Input: part model. Units: mm. Frame: model coordinates. Face numbers are marked on the shaded views. A direction names the side the tool comes from. Coordinates: 2 decimals unless noted, no trailing zeros. Loops run counter-clockwise (first coordinate to the right, second up) from the corner with the lowest first, then second, coordinate; pieces in that order, holes last.
(1) Contact query for flat-ended pins moving along their axis: P1, Ø1.5, axis at y = -12.5, z = 2, coming from the -X side; P2, Ø1, axis at y = 3, z = 1.5, coming from the -X side. Output: stop coordinate, or through.
(2) Mould query, pull axis X, two halves, no side actions, for the marked faces 1, 2, 3 and 4. Classes: released by +X, released by -X, zero draft, split by the parting line, or undercut.
(3) Section A-A, the plane z = 0.8. Return loops of the section in (x, y), then the cut area to 3 significant figures.
(4) Set-up query: the marked faces 5 and 6. Return all of +Z, -Z, +X, -X, +Y, -Y with unobstructed straight access to the full face (end or side cutting, diameter ignored); none if empty.
(5) Line query: L1, parallel to X at y = -7, z = 1.85; L2, parallel to Z at x = 1.25, y = 5.25; L3, parallel to X at y = -8.5, z = 1.9. Output: solid intervals per line, ascending.
(6) Section B-B, the plane x = 0. Return loops of the section in (y, z).
(7) Section C-C, the plane z = 2.05. Return loops of the section in (x, y), then the cut area to 3 significant figures.
(8) Section D-D, the plane y = -11.25. Return loops of the section in (x, z), then the cut area to 4 significant figures.
```python
from build123d import *

# Parameters (mm, degrees)
F1_DEPTH    = 3
F3_DEPTH    = 1.5
F4_R        = 3.5
F5_DEPTH    = 1.5
F6_T1_DEPTH = 2.7420993995
F7_R        = 5


# Not quite as in the source:
# - a fillet or chamfer that OpenCascade refuses, or shapes differently, is made with other operations: its cross-section is extruded or revolved along the edge and cut away or added


with BuildPart() as f1:
    # F0 (on Top) → F1 (new body)
    with BuildSketch(Plane.XY):
        with BuildLine():
            ThreePointArc((2.5, -7.0710678119), (6.123724357, -4.3301270189), (7.5, 0))
            ThreePointArc((7.5, 0), (-4.3301270189, 6.123724357), (-2.5, -7.0710678119))
            Line((-2.5, -7.0710678119), (2.5, -7.0710678119))
        make_face()
        with BuildLine():
            Line((2.5, -7.0710678119), (-2.5, -7.0710678119))
            ThreePointArc((-2.5, -7.0710678119), (0, -7.5), (2.5, -7.0710678119))
        make_face()
        with BuildLine():
            ThreePointArc((2.5, -7.0710678119), (0, -7.5), (-2.5, -7.0710678119))
            Line((-2.5, -7.0710678119), (-2.5, -16.4693647414))
            Line((-2.5, -16.4693647414), (2.5, -16.4693647414))
            Line((2.5, -16.4693647414), (2.5, -7.0710678119))
        make_face()
    extrude(amount=F1_DEPTH)

    # F2 (on face) → F3 (cut)
    with BuildSketch(Plane.XY.offset(3)):
        with BuildLine():
            ThreePointArc((1.45, -5.9251582257), (4.79869774, -3.7659660115), (6.1, 0))
            ThreePointArc((6.1, 0), (-3.7659660115, 4.79869774), (-1.45, -5.9251582257))
            Line((-1.45, -5.9251582257), (1.45, -5.9251582257))
        make_face()
        with BuildLine():
            Line((1.45, -5.9251582257), (-1.45, -5.9251582257))
            ThreePointArc((-1.45, -5.9251582257), (0, -6.1), (1.45, -5.9251582257))
        make_face()
        with BuildLine():
            ThreePointArc((1.45, -5.9251582257), (0, -6.1), (-1.45, -5.9251582257))
            Line((-1.45, -5.9251582257), (-1.45, -16.4693647414))
            Line((-1.45, -16.4693647414), (1.45, -16.4693647414))
            Line((1.45, -16.4693647414), (1.45, -5.9251582257))
        make_face()
    extrude(amount=-F3_DEPTH, mode=Mode.SUBTRACT)

    # F4 (on face) → F5 (cut, through all)
    with BuildSketch(Plane.XY.offset(1.5)):
        Circle(F4_R)
    extrude(amount=-F5_DEPTH, mode=Mode.SUBTRACT)

    # F6: chamfer of 0.5 on 2 edges, made by hand

    # F6_s2 → F6_t1 (cut)
    with BuildSketch(Plane.XY.offset(1.5)):
        with BuildLine():
            Line((1.4382509018, -6.4218590468), (1.9014892015, -5.7837185114))
            Line((1.9014892015, -5.7837185114), (1.8983912669, -5.7742104726))
            ThreePointArc((1.8983912669, -5.7742104726), (1.6758695773, -5.854874991), (1.4476229508, -5.9154448516))
            Line((1.4476229508, -5.9154448516), (1.44, -5.9251582257))
            ThreePointArc((1.44, -5.9251582257), (1.44, -6.1735086363), (1.4282509018, -6.4218590468))
            Line((1.4282509018, -6.4218590468), (1.4382509018, -6.4218590468))
        make_face()
        with BuildLine():
            Line((-1.4382509018, -6.4218590468), (-1.9014892015, -5.7837185114))
            Line((-1.9014892015, -5.7837185114), (-1.8983912669, -5.7742104726))
            ThreePointArc((-1.8983912669, -5.7742104726), (-1.6758695773, -5.854874991), (-1.4476229508, -5.9154448516))
            Line((-1.4476229508, -5.9154448516), (-1.44, -5.9251582257))
            ThreePointArc((-1.44, -5.9251582257), (-1.44, -6.1735086363), (-1.4282509018, -6.4218590468))
            Line((-1.4282509018, -6.4218590468), (-1.4382509018, -6.4218590468))
        make_face()
    extrude(amount=F6_T1_DEPTH, mode=Mode.SUBTRACT)

    # F7
    f7_edges = [f1.edges().sort_by_distance(p)[0] for p in [
        (-2.5, -7.071068, 1.5),
        (2.5, -7.071068, 1.5),
    ]]
    fillet(f7_edges, radius=F7_R)


solid = f1.part
```
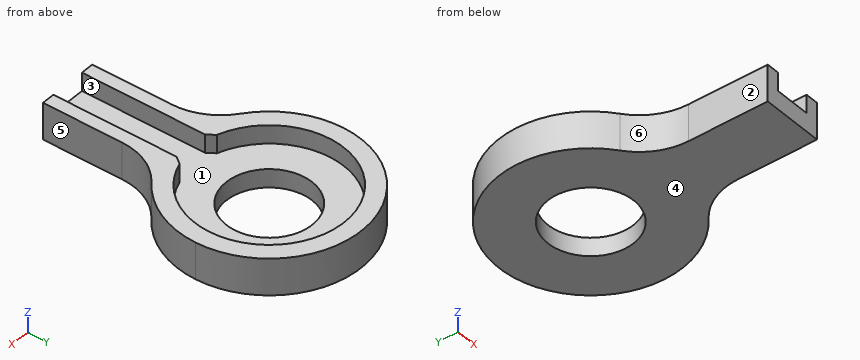
Report:
1. P1: stops at x = -2.5
1. P2: stops at x = -7.07
2. face 1: undercut
2. face 2: released by -X
2. face 3: undercut
2. face 4: zero draft
3. outline: (-4.5, -6) arc R5 cw to (-2.5, -10) - (-2.5, -16.47) - (2.5, -16.47) - (2.5, -10) arc R5 cw to (4.5, -6) arc R7.5 ccw (long way) to start; hole circle Ø7 at (0, 0)
3. area: 186 mm2
4. face 5: +Z, -Z, +X, -Y
4. face 6: +Z, -Z, -X, -Y
5. L1: x = -3.5 to -1.45, 1.45 to 3.5
5. L2: z = 0 to 1.5
5. L3: x = -2.73 to -1.45, 1.45 to 2.73
6. outline: (-16.47, 0) - (-3.5, 0) - (-3.5, 1.5) - (-16.47, 1.5) - close; (3.5, 0) - (7.5, 0) - (7.5, 3) - (6.1, 3) - (6.1, 1.5) - (3.5, 1.5) - close
7. outline: (-4.5, -6) arc R5 cw to (-2.5, -10) - (-2.5, -16.47) - (-1.45, -16.47) - (-1.45, -6.41) - (-1.89, -5.8) arc R6.1 cw (long way) to (1.89, -5.8) - (1.45, -6.41) - (1.45, -16.47) - (2.5, -16.47) - (2.5, -10) arc R5 cw to (4.5, -6) arc R7.5 ccw (long way) to start
7. area: 77.3 mm2
8. outline: (-2.5, 0) - (2.5, 0) - (2.5, 3) - (1.45, 3) - (1.45, 1.5) - (-1.45, 1.5) - (-1.45, 3) - (-2.5, 3) - close
8. area: 10.65 mm2
